Geometry check sheet. Reference: the model listing, model coordinates, mm. A direction names the side the tool comes from. Round coordinates to 2 decimals unless told otherwise and drop trailing zeros. Write each loop counter-clockwise with the first axis right and the second up, starting at its lowest first coordinate (ties: lowest second). Pieces come first, ordered by that corner, then holes. Notation, with made-up numbers: M -16,-1 L 15,-1 A25 cw 15,36 Z; hole C 51.25,52 d8. An arc over 180 degrees is marked long. Put each result on its own line as item: value. Start each with the question number.
(1) Section check A-A on y = -11. Record the cut outline in (x, z) (3 decimals).
(2) Section check D-D on x = -11.5. Record the cut outline in (y, z).
(3) Section check B-B on x = -25.4. Record the cut outline in (y, z), then the cut area to 3 significant figures.
(4) Mould release check, pull along X, two halves, no side actions. Record for faces 1 (the cylindrical face through (-26.68, 0.78, 48.79)), 2 (the flat face through (-31, 1.588, 52)), 3 (the flat face through (-53.975, -6, 52)): pulls with the +X half, pulls with the -X half, needs draft (parallel to the pull), parting line crosses it, or undercut.
(5) Material ranges on probe 1 along Z at (x, y) = (-25.4, 1.25); probe 2 along X at (y, z) = (0.45, 50.8) (3 decimals); probe 3 along X at (y, z) = (-2, 81) (3 decimals), recorded low to high.
(6) Section check C-C on z = 50.8. Record the cut outline in (x, y) (1 decimal), then the cut area to 3 significant figures.
(7) Gauge pin test, flat end, axial feed: pin 1 (6 mm diameter, centred on x = -37.5, z = 72.5, fed in from -Y). Record the tip position at first contact, or that the pin passes through.
(8) Tool access check on faces 4 (the flat face through (3.175, -6, 52)), 5 (the flat face through (-31, 0, 52)). Record the directions out of +Z, -Z, +X, -X, +Y, -Y that give a thin tool (end or side, any length) a straight path to the whole face; none if there is none.
Autodesk Inventor part; units mm, degrees
ref_plane "YZ Plane" through (0, 0, 0) normal (1, 0, 0) x (0, 1, 0)
ref_plane "XZ Plane" through (0, 0, 0) normal (0, 1, 0) x (-1, 0, 0)
ref_plane "XY Plane" through (0, 0, 0) normal (0, 0, 1) x (1, 0, 0)
sketch "Sketch1" plane through (0, 0, 0) normal (0, 1, 0) x (-1, 0, 0)
  line L0 (0, 0) -> (50.8, 0)
  line L1 (50.8, 0) -> (50.8, 101.6)
  line L2 (50.8, 101.6) -> (0, 101.6)
  line L3 (0, 101.6) -> (0, 0)
  line L4 (50.8, 101.6) -> (53.975, 101.6)
  line L5 (53.975, 101.6) -> (53.975, 0)
  line L6 (53.975, 0) -> (50.8, 0)
  line L7 (50.8, 0) -> (50.8, 101.6)
  line L8 (0, 101.6) -> (-3.175, 101.6)
  line L9 (-3.175, 101.6) -> (-3.175, 0)
  line L10 (-3.175, 0) -> (0, 0)
  line L11 (0, 0) -> (0, 101.6)
  circle A0 centre (25.4, 50.8) radius 2.3813
  line L12 (50.8, 53.1813) -> (0, 53.1813)
  line L13 (0, 53.1813) -> (0, 48.4188)
  line L14 (0, 48.4188) -> (50.8, 48.4188)
  line L15 (50.8, 48.4188) -> (50.8, 53.1813)
  line L16 (27.7813, 101.6) -> (23.0188, 101.6)
  line L17 (23.0188, 101.6) -> (23.0188, 0)
  line L18 (23.0188, 0) -> (27.7813, 0)
  line L19 (27.7813, 0) -> (27.7813, 101.6)
  line L20 (27.7812, 65.8812) -> (23.0187, 65.8812)
  line L21 (23.0187, 65.8812) -> (23.0187, 59.5312)
  line L22 (23.0187, 59.5312) -> (27.7812, 59.5312)
  line L23 (27.7812, 59.5312) -> (27.7812, 65.8812)
  line L24 (40.4812, 53.1813) -> (34.1313, 53.1813)
  line L25 (34.1313, 53.1813) -> (34.1313, 48.4188)
  line L26 (34.1313, 48.4188) -> (40.4812, 48.4188)
  line L27 (40.4812, 48.4188) -> (40.4812, 53.1813)
  line L28 (27.7812, 42.0688) -> (23.0187, 42.0688)
  line L29 (23.0187, 42.0688) -> (23.0188, 35.7188)
  line L30 (23.0188, 35.7188) -> (27.7812, 35.7188)
  line L31 (27.7812, 35.7188) -> (27.7812, 42.0688)
  line L32 (16.6687, 53.1813) -> (10.3187, 53.1813)
  line L33 (10.3187, 53.1813) -> (10.3188, 48.4188)
  line L34 (10.3188, 48.4188) -> (16.6688, 48.4188)
  line L35 (16.6688, 48.4188) -> (16.6687, 53.1813)
  point P0 (0, 50.8)
  point P1 (25.4, 53.1813)
  point P2 (25.4, 35.7188)
  point P3 (25.4, 42.0688)
  dimension "d0" = 50.8
  dimension "d1" = 101.6
  dimension "d2" = 3.175
  dimension "d3" = 101.6
  dimension "d4" = 3.175
  dimension "d5" = 101.6
  dimension "d6" = 4.7625
  dimension "d7" = 25.4
  dimension "d8" = 50.8
  dimension "d9" = 4.7625
  dimension "d10" = 4.7625
  dimension "d11" = 2.3813
  dimension "d12" = 2.3813
  dimension "d13" = 6.35
  dimension "d14" = 6.35
  dimension "d15" = 6.35
  dimension "d16" = 6.35
  dimension "d17" = 6.35
  dimension "d18" = 6.35
  dimension "d19" = 6.35
  dimension "d20" = 6.35
extrude "Extrusion1" add sketch "Sketch1" along normal blind 1.5875 contours L3 L14 L17 L0 | L17 L30 L19 L0 | L3 L12 L33 L14 | L19 L14 L1 L0 | L3 L2 L17 L12 | L17 L14 L19 L28 | L35 L12 L17 L14 | L14 L27 L12 L1 | L17 A0 L14 | L2 L19 L20 L17 | L12 L19 L2 L1 | L19 L12 L25 L14 | L14 A0 L19 | L17 L12 A0 | L17 L22 L19 L12 | A0 L12 L19
extrude "Extrusion2" add sketch "Sketch1" along normal blind 1.5875 and the other way blind 12.7 contours L10 L9 L8 L3 | L1 L4 L5 L6
equation "\"d12\" = 0.5 * d6"
equation "\"d15\" = d14"
equation "\"d16\" = d15"
properties part number "Guide for 2in box tube"
Answers follow:
1. outline: M -53.975,0 L -50.8,0 L -50.8,101.6 L -53.975,101.6 Z; M 0,0 L 3.175,0 L 3.175,101.6 L 0,101.6 Z
2. outline: M 0,0 L 1.59,0 L 1.59,48.42 L 0,48.42 Z; M 0,53.18 L 1.59,53.18 L 1.59,101.6 L 0,101.6 Z
3. outline: M 0,0 L 1.59,0 L 1.59,35.72 L 0,35.72 Z; M 0,42.07 L 1.59,42.07 L 1.59,48.42 L 0,48.42 Z; M 0,53.18 L 1.59,53.18 L 1.59,59.53 L 0,59.53 Z; M 0,65.88 L 1.59,65.88 L 1.59,101.6 L 0,101.6 Z
3. area: 134 mm^2
4. face 1: undercut
4. face 2: needs draft
4. face 3: pulls with the -X half
5. probe 1: z = 0 to 35.72, 42.07 to 48.42, 53.18 to 59.53, 65.88 to 101.6
5. probe 2: x = -53.975 to -40.481, -34.131 to -27.781, -23.019 to -16.669, -10.319 to 3.175
5. probe 3: x = -53.975 to -50.8, 0 to 3.175
6. outline: M -54,-12.7 L -50.8,-12.7 L -50.8,0 L -40.5,0 L -40.5,1.6 L -54,1.6 Z; M -34.1,0 L -27.8,0 L -27.8,1.6 L -34.1,1.6 Z; M -23,0 L -16.7,0 L -16.7,1.6 L -23,1.6 Z; M -10.3,0 L 0,0 L 0,-12.7 L 3.2,-12.7 L 3.2,1.6 L -10.3,1.6 Z
6. area: 144 mm^2
7. pin 1: stops at y = 0
8. face 4: +Z, -Z, +X, +Y, -Y
8. face 5: +Z, -Z, -Y
